Input: dimensioned drawing with shaded views. Units: mm. Origin: part minimum x, y, z. A direction names the side the tool comes from. Round coordinates to 2 decimals unless told otherwise and drop trailing zeros. Loops run counter-clockwise (first coordinate to the right, second up) from the corner with the lowest first, then second, coordinate; pieces in that order, holes last. Notation, with made-up numbers: M -4,82.5 L 48,82.5 A21 ccw 48,121.5 Z; hole C 9.5,-21 d2. An arc over 180 degrees is marked long. One line per item, written item: value.
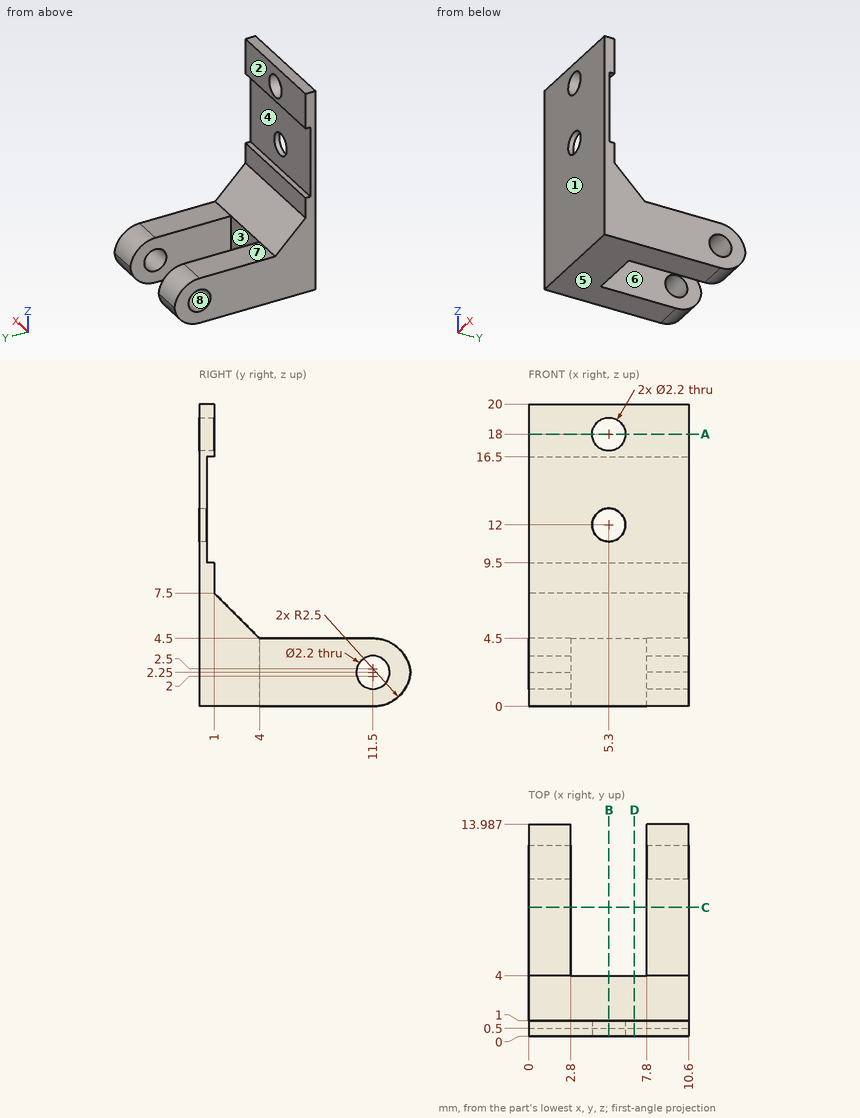
1. Section query D-D (x = 7). Return the cut outline in (y, z).
Report:
outline: M 0,0 L 4,0 L 4,4.5 L 1,7.5 L 1,9.5 L 0.5,9.5 L 0.5,16.5 L 1,16.5 L 1,20 L 0,20 Z
2. Pull-direction query (Z, two-part tool) for the marked faces 6, 7 and 8; classes: released by +Z, released by -Z, zero draft, split by the parting line, or undercut.
Report:
face 6: zero draft
face 7: released by +Z
face 8: undercut
3. Ray query, line 1 (X direction, y = 0.45, z = 12); line 2 (X direction, y = 13, z = 3.25); line 3 (Y direction, x = 9.85, z = 2.25). Return the intervals inside material, ascending. Write a range as [from, to].
Report:
line 1: x = [0, 4.2], [6.4, 10.6]
line 2: x = [0, 2.8], [7.8, 10.6]
line 3: y = [0, 10.4], [12.6, 13.99]
4. Section query A-A (z = 18). Return the cut outline in (x, y).
Report:
outline: M 0,0 L 4.2,0 L 4.2,1 L 0,1 Z; M 6.4,0 L 10.6,0 L 10.6,1 L 6.4,1 Z
5. Section query C-C (y = 8.5). Return the cut outline in (x, z), and give its area (3 significant figures).
Report:
outline: M 0,0 L 2.8,0 L 2.8,4.5 L 0,4.5 Z; M 7.8,0 L 10.6,0 L 10.6,4.5 L 7.8,4.5 Z
area: 25.2 mm2
6. Section query B-B (x = 5.3). Return the cut outline in (y, z), and give its area (3 significant figures).
Report:
outline: M 0,0 L 4,0 L 4,4.5 L 1,7.5 L 1,9.5 L 0.5,9.5 L 0.5,10.9 L 0,10.9 Z; M 0,13.1 L 0.5,13.1 L 0.5,16.5 L 1,16.5 L 1,16.9 L 0,16.9 Z; M 0,19.1 L 1,19.1 L 1,20 L 0,20 Z
area: 31.2 mm2
7. Reachability of the marked faces 1, 2, 3, 4 and 5 from +Z, -Z, +X, -X, +Y, -Y: full face, straight path, thin tool, end or side. Return the list, or none.
Report:
face 1: +Z, -Z, +X, -X, -Y
face 2: +Z, +X, -X, +Y
face 3: +Z, -Z, +Y
face 4: +X, -X, +Y
face 5: -Z, +X, -X, +Y, -Y
8. Pin query (flat end, axial travel): pin 1 (2 mm diameter, centred on x = 3, z = 13.5, fed in from +Y); pin 2 (5 mm diameter, centred on x = 5, z = 1, fed in from +Y); pin 3 (0.6 mm diameter, centred on x = 6, z = 8, fed in from +Y). Return the tip coordinate at first contact, or that it passes through.
Report:
pin 1: stops at y = 0.5
pin 2: stops at y = 13.98
pin 3: stops at y = 1
